Drawing for the job (mm, zero at the part's lowest x, y, z). A direction names the side the tool comes from. Coordinates: 2 decimals unless noted, no trailing zeros. Loops run counter-clockwise (first coordinate to the right, second up) from the corner with the lowest first, then second, coordinate; pieces in that order, holes last.
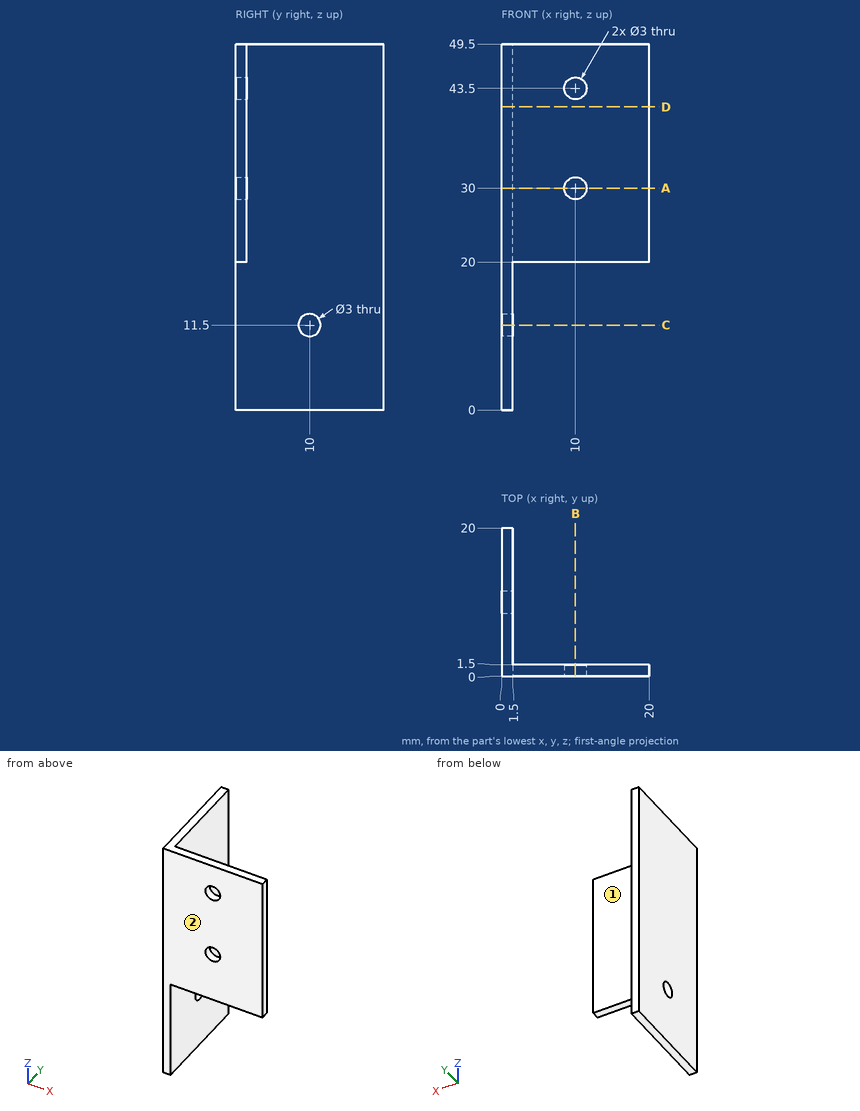
Q1. Saw through at D-D (z = 41). List the corners of the cut face in (x, y), plus the area to 4 significant figures.
Q2. Saw through at A-A (z = 30). List the corners of the cut face in (x, y).
Q3. Drop flat-ended pins along their axis: P1, Ø10, axis at y = 15, z = 30.5, coming from the +X side; P2, Ø2.5, axis at y = 10, z = 11.5, coming from the +X side; P3, Ø4, axis at x = 10, z = 43.5, coming from the +Y side. Give the stop position or say it passes through.
Q4. Probe line 1 (Z direction, x = 10, y = 0.3); line 2 (X direction, y = 15.75, z = 23); line 3 (Y direction, x = 0.95, z = 11.5). List the from-to ranges inside material, lowest first.
Q5. Tool access for the marked faces 1 and 2: list every direction of +Z, -Z, +X, -X, +Y, -Y with a clear straight run to the whole face (end or side of a thin tool).
Q6. Saw through at C-C (z = 11.5). List the corners of the cut face in (x, y).
Q7. Saw through at B-B (x = 10). List the corners of the cut face in (y, z), plus the area to 4 significant figures.
Checked values:
1. outline: (0, 0) - (20, 0) - (20, 1.5) - (1.5, 1.5) - (1.5, 20) - (0, 20) - close
1. area: 57.75 mm2
2. outline: (0, 0) - (8.5, 0) - (8.5, 1.5) - (1.5, 1.5) - (1.5, 20) - (0, 20) - close; (11.5, 0) - (20, 0) - (20, 1.5) - (11.5, 1.5) - close
3. P1: stops at x = 1.5
3. P2: passes through
3. P3: stops at y = 1.5
4. line 1: z = 20 to 28.5, 31.5 to 42, 45 to 49.5
4. line 2: x = 0 to 1.5
4. line 3: y = 0 to 8.5, 11.5 to 20
5. face 1: +Z, -Z, +X, +Y
5. face 2: +Z, -Z, +X, -X, -Y
6. outline: (0, 0) - (1.5, 0) - (1.5, 8.5) - (0, 8.5) - close; (0, 11.5) - (1.5, 11.5) - (1.5, 20) - (0, 20) - close
7. outline: (0, 20) - (1.5, 20) - (1.5, 28.5) - (0, 28.5) - close; (0, 31.5) - (1.5, 31.5) - (1.5, 42) - (0, 42) - close; (0, 45) - (1.5, 45) - (1.5, 49.5) - (0, 49.5) - close
7. area: 35.25 mm2
